Input: dimensioned drawing with shaded views. Units: mm. Origin: part minimum x, y, z. Round coordinates to 2 decimals unless told otherwise and drop trailing zeros. Loops run counter-clockwise (first coordinate to the right, second up) from the corner with the lowest first, then second, coordinate; pieces in that order, holes last. Notation, with made-up numbers: M -10,-22.5 L 3,-22.5 A8 cw 3,-15.5 Z; hole C -21,52.5 d3. An arc over 180 degrees is marked long. Put each result on its own line as item: value. Start each with the question number.
1) Section A-A on x = 22. Output: boundary loops of the cut face in (y, z), plus the area to 3 significant figures.
2) Line query: probe 1 along Y at (x, z) = (22, 12.75); probe 2 along X at (y, z) = (28, 7); probe 3 along X at (y, z) = (12.5, 2). Output: solid intervals per line, ascending.
3) Section B-B on z = 6.75. Output: boundary loops of the cut face in (x, y).
4) Section C-C on y = 27.5. Output: boundary loops of the cut face in (x, z).
5) Draft query along Z for the marked faces 1, 2 and 3. Return one class per face: +Z half, -Z half, draft (parallel to the pull), parting line (faces both ways), or undercut.
6) Section D-D on y = 12.75. Output: boundary loops of the cut face in (x, z).
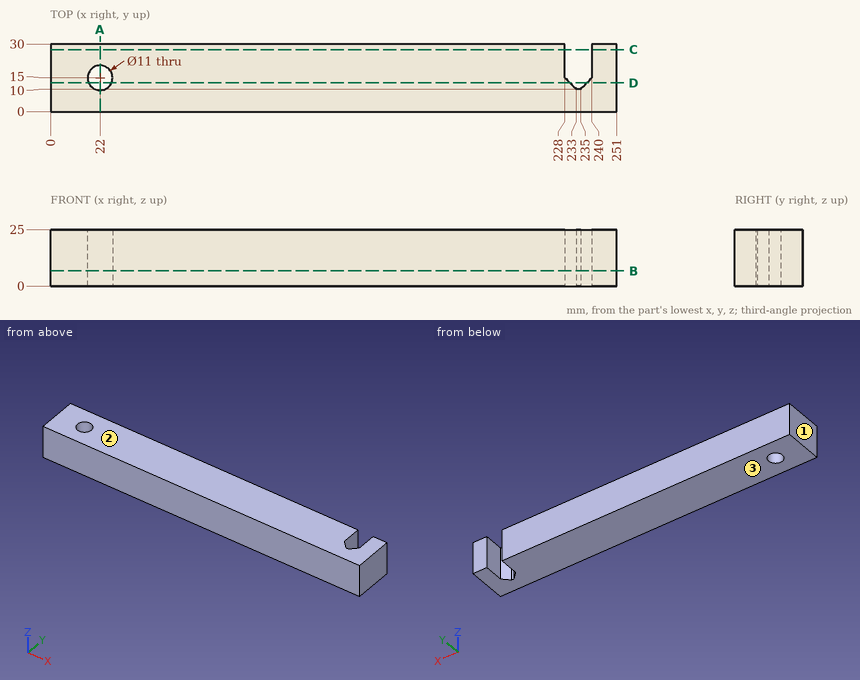
Geometry results:
1. outline: M 0,0 L 9.5,0 L 9.5,25 L 0,25 Z; M 20.5,0 L 30,0 L 30,25 L 20.5,25 Z
1. area: 475 mm²
2. probe 1: y = 0 to 9.5, 20.5 to 30
2. probe 2: x = 0 to 228, 240 to 251
2. probe 3: x = 0 to 17.1, 26.9 to 230.5, 237.5 to 251
3. outline: M 0,0 L 251,0 L 251,30 L 240,30 L 240,15 L 235,10 L 233,10 L 228,15 L 228,30 L 0,30 Z; hole C 22,15 d11
4. outline: M 0,0 L 228,0 L 228,25 L 0,25 Z; M 240,0 L 251,0 L 251,25 L 240,25 Z
5. face 1: draft
5. face 2: +Z half
5. face 3: -Z half
6. outline: M 0,0 L 16.98,0 L 16.98,25 L 0,25 Z; M 27.02,0 L 230.25,0 L 230.25,25 L 27.02,25 Z; M 237.75,0 L 251,0 L 251,25 L 237.75,25 Z
